Autodesk Inventor part; units mm, degrees
ref_plane "Plano de trabalho1" through (0, 28, 40) normal (1, 0, 0) x (0, 0, -1)
ref_plane "YZ Plane" through (0, 0, 0) normal (1, 0, 0) x (0, 1, 0)
ref_plane "XZ Plane" through (0, 0, 0) normal (0, 1, 0) x (-1, 0, 0)
sketch "Esboço1" plane through (0, 0, 0) normal (0, 1, 0) x (-1, 0, 0)
  line L0 (-50, 50) -> (50, 50)
  line L1 (50, 50) -> (50, -50)
  line L2 (50, -50) -> (-50, -50)
  line L3 (-50, -50) -> (-50, 50)
  line L4 (-50, 50) -> (50, -50) construction
  line L5 (50, 50) -> (-50, -50) construction
  point P0 (0, 0)
  dimension "d0" = 100
  dimension "d1" = 100
extrude "Extrusão1" add sketch "Esboço1" along normal blind 28
sketch "Esboço3" plane through (0, 28, 0) normal (0, 1, 0) x (1, 0, 0)
  line L0 (50, 50) -> (-50, 50)
  line L1 (-40, 50) -> (40, 50)
  line L2 (-40, 50) -> (-40, -40)
  line L3 (-40, -40) -> (40, -40)
  line L4 (40, -40) -> (40, 50)
  point P0 (0, 0)
  point P1 (0, 50)
  dimension "d5" = 80
  dimension "d6" = 90
extrude "Extrusão2" cut sketch "Esboço3" against normal blind 28 keep common part
shell "Casca2" thickness 2.5 removed faces 1 at (-13.3333, 28, 10)
ref_plane "Plano de trabalho1" through (0, 28, 40) normal (1, 0, 0) x (0, 0, -1)
sketch "Esboço4" plane through (40, 28, 40) normal (1, 0, 0) x (0, 0, -1)
  circle A0 centre (76.5, -14.5) radius 17.5
  line L0 (90, -28) -> (90, 0)
  line L1 (0, -28) -> (90, -28)
  circle A1 centre (76.5, -14.5) radius 16.1
  circle A2 centre (76.5, -14.5) radius 11
  line L2 (87.5, -25.5) -> (87.5, 0)
  line L3 (2.5, -25.5) -> (87.5, -25.5)
  line L4 (90, 0) -> (66.702, 0)
  line L5 (90, 0) -> (90, -28)
  line L6 (90, -28) -> (87.6355, -28)
  point P0 (40, -28)
  point P1 (90, -25.6355)
  point P2 (90, -3.3645)
  point P3 (86.298, 0)
  dimension "d11" = 35
  dimension "d14" = 32.2
  dimension "d15" = 22
extrude "Extrusão3" cut sketch "Esboço4" against normal blind 12
sketch "Esboço5" plane through (28, 28, 40) normal (1, 0, 0) x (0, 0, -1)
  arc A0 (66.702, 0) -> (65.3645, -28) centre (76.5, -14.5) ccw
  arc A1 (65.3023, 2.0714) -> (63.7737, -29.9286) centre (76.5, -14.5) ccw
  line L0 (65.3645, -28) -> (61.7436, -28)
  line L1 (90, -28) -> (0, -28)
  line L2 (66.702, 0) -> (62.725, 0)
  point P0 (40, -28)
  dimension "d18" = 2.5
extrude "Extrusão4" add sketch "Esboço5" along normal up to surface (12 mm away)
sketch "Esboço6" plane through (28, 28, 40) normal (-1, 0, 0) x (0, 0, 1)
  arc A0 (-59.7967, -25.5) -> (-62.725, 0) centre (-76.5, -14.5) ccw
  line L0 (-66.702, 0) -> (-62.725, 0)
  line L1 (-87.5, -25.5) -> (-87.5, 0)
  line L2 (-87.5, -25.5) -> (-59.7967, -25.5)
  line L3 (-87.5, 0) -> (-66.702, 0)
  point P0 (-40, -28)
extrude "Extrusão5" add sketch "Esboço6" along normal blind 8
sketch "Esboço7" plane through (20, 28, 40) normal (-1, 0, 0) x (0, 0, 1)
  arc A0 (-59.7967, -25.5) -> (-62.725, 0) centre (-76.5, -14.5) ccw
  circle A1 centre (-76.5, -14.5) radius 11
  point P0 (-40, -28)
  dimension "d23" = 22
extrude "Extrusão6" cut sketch "Esboço7" against normal blind 6.9
chamfer "Chanfro1" distance 7 angle 45 1 edges at (20, 15.7817, -16.6306)
sketch "Esboço8" plane through (28, 28, 40) normal (1, 0, 0) x (0, 0, -1)
  arc A0 (66.702, 0) -> (65.3645, -28) centre (76.5, -14.5) ccw
  circle A1 centre (76.5, -14.5) radius 7
  point P0 (40, -28)
  dimension "d29" = 14
extrude "Extrusão7" cut sketch "Esboço8" against normal blind 8
mirror "Espelhar1" about plane through (0, 28, 40) normal (1, 0, 0) of "Extrusão3", "Extrusão4", "Extrusão5", "Extrusão6", "Chanfro1", "Extrusão7"
properties part number "Base"
Geometry check sheet. Reference: the model listing, model coordinates, mm. A direction names the side the tool comes from. Round coordinates to 2 decimals unless told otherwise and drop trailing zeros. Write each loop counter-clockwise with the first axis right and the second up, starting at its lowest first coordinate (ties: lowest second). Pieces come first, ordered by that corner, then holes. Notation, with made-up numbers: (74.25, -12) -> (120.25, -12) arc R32 cw to (120.25, 26) -> close; hole circle Ø4 at (79, 53). An arc over 180 degrees is marked (long way). Put each result on its own line as item: value.
1) Release check for a two-part mould opening along Y. For faces 6 (the face through (1, 0, -4)), 7 (the face through (27.46, 7.29, -39.73)), 8 (the face through (0, 14, -50)) record: pulls with the +Y half, pulls with the -Y half, needs draft (parallel to the pull), parting line crosses it, or undercut.
Recorded:
face 6: pulls with the -Y half
face 7: undercut
face 8: needs draft
2) Cross-section at B-B, the plane x = 12.5. Enter the section's corners in (y, z).
Recorded:
outline: (0, -50) -> (28, -50) -> (28, -47.5) -> (2.5, -47.5) -> (2.5, 37.5) -> (28, 37.5) -> (28, 40) -> (0, 40) -> close
3) Access from +Z, -Z, +X, -X, +Y, -Y to the whole of each face (thin tool, end or side, straight path). Record for faces 1 (the face through (28, 20, -31)), 2 (the face through (-28, 20.4, -34.3)), 3 (the face through (-40, 14, 6)), 4 (the face through (-20, 23, -30)), 5 (the face through (-20.44, 18.25, -23.93)).
Recorded:
face 1: -Z, +X
face 2: -Z, -X
face 3: +Z, -Z, -X, +Y, -Y
face 4: +Y
face 5: none
4) Thickness scan on probe 1 along Z at (x, y) = (-12.5, 17.25); probe 2 along Z at (x, y) = (33.5, 14); probe 3 along Y at (x, z) = (-22.5, -36.5). Record the ranges inside material, lowest first. Write a range as from..to.
Recorded:
probe 1: z = -50..-47.5, 37.5..40
probe 2: z = -19.01..-16.51, 37.5..40
probe 3: y = 0..2.5, 24.5..28
5) Depth check by flat-ended pin: P1, Ø8.5, axis at y = 16.5, z = -37, coming from the +X side; P2, Ø22.5, axis at x = 16, z = -8.5, coming from the +Y side; P3, Ø3.5, axis at y = 9, z = -39.5, coming from the -X side. Enter the tip coordinate at first touch or a pass-through.
Recorded:
P1: stops at x = 28
P2: stops at y = 2.5
P3: stops at x = -28
6) Cross-section at C-C, the plane x = 24. Enter the section's corners in (y, z), plus the area to 3 significant figures.
Recorded:
outline: (0, -50) -> (28, -50) -> (28, -47.5) -> (26.46, -47.5) arc R17 ccw to (28, -45.37) -> (28, -27.63) arc R17 ccw to (2.5, -23.54) -> (2.5, 37.5) -> (28, 37.5) -> (28, 40) -> (0, 40) -> close; hole circle Ø22 at (13.5, -36.5)
area: 636 mm2
7) Cross-section at A-A, the plane z = -8.5. Enter the section's corners in (x, y), plus the area to 4 significant figures.
Recorded:
outline: (-40, 0) -> (40, 0) -> (40, 28) -> (37.5, 28) -> (37.5, 2.5) -> (-37.5, 2.5) -> (-37.5, 28) -> (-40, 28) -> close
area: 327.5 mm2
